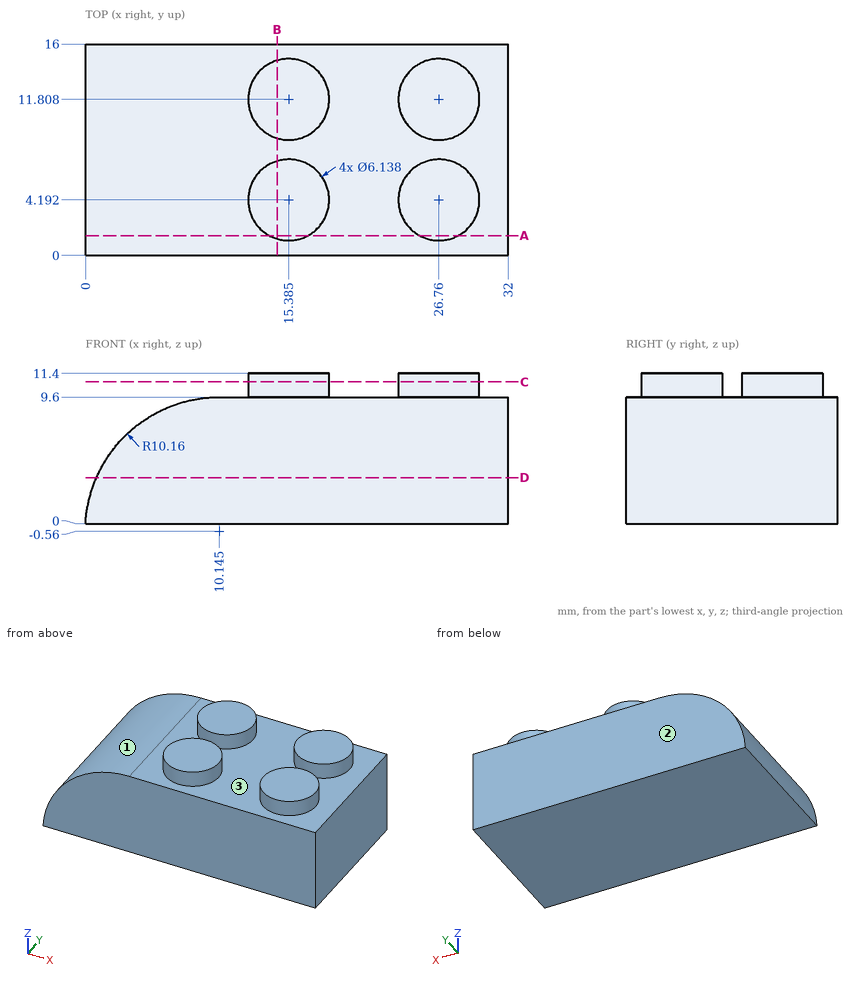
Design review of the part shown in the three views and the two pictorial views. Dimensions are in mm from the part's minimum x, y and z. Coordinates: 2 decimals unless noted, no trailing zeros. Write each loop counter-clockwise with the first axis right and the second up, starting at its lowest first coordinate (ties: lowest second). Pieces come first, ordered by that corner, then holes. Notation, with made-up numbers: (27, 87.25) -> (36, 87.25) arc R25 ccw to (36, 108.25) -> close; hole circle Ø10 at (-35, 82). An arc over 180 degrees is marked (long way). Answer in a Markdown table with one row per item.
1. Wall thickness on probe 1 along Z at (x, y) = (30, 7.5); probe 2 along Y at (x, z) = (26, 10) (1 decimal); probe 3 along X at (y, z) = (8.75, 6) (1 decimal): over which ranges is each line inside the solid? List them lowest first. Write a range as [from, to].
Answers below:
| item | result |
|---|---|
| probe 1 | z = [0, 9.6] |
| probe 2 | y = [1.2, 7.2], [8.8, 14.8] |
| probe 3 | x = [2.4, 32] |
2. Draft analysis for pull direction X (two halves, no side actions). For the marked faces 1, 2 and 3, state which applies: +X half, -X half, draft (parallel to the pull), parting line (faces both ways), or undercut.
Answers below:
| item | result |
|---|---|
| face 1 | -X half |
| face 2 | draft |
| face 3 | undercut |
3. We need section C-C, the plane z = 10.75. State the section outline as (x, y) points (1 decimal).
Answers below:
| item | result |
|---|---|
| outline | circle Ø6.1 at (15.4, 4.2); circle Ø6.1 at (15.4, 11.8); circle Ø6.1 at (26.8, 4.2); circle Ø6.1 at (26.8, 11.8) |
4. We need section D-D, the plane z = 3.5. State the section outline as (x, y) points, and give its area (3 significant figures).
Answers below:
| item | result |
|---|---|
| outline | (0.83, 0) -> (32, 0) -> (32, 16) -> (0.83, 16) -> close |
| area | 499 mm^2 |
5. We need section B-B, the plane x = 14.5. State the section outline as (y, z) points.
Answers below:
| item | result |
|---|---|
| outline | (0, 0) -> (16, 0) -> (16, 9.6) -> (14.75, 9.6) -> (14.75, 11.4) -> (8.87, 11.4) -> (8.87, 9.6) -> (7.13, 9.6) -> (7.13, 11.4) -> (1.25, 11.4) -> (1.25, 9.6) -> (0, 9.6) -> close |
6. We need section A-A, the plane y = 1.5. State the section outline as (x, z) points (1 decimal), and give its area (3 significant figures).
Answers below:
| item | result |
|---|---|
| outline | (0, 0) -> (32, 0) -> (32, 9.6) -> (28.2, 9.6) -> (28.2, 11.4) -> (25.3, 11.4) -> (25.3, 9.6) -> (16.9, 9.6) -> (16.9, 11.4) -> (13.9, 11.4) -> (13.9, 9.6) -> (10.1, 9.6) arc R10.2 ccw to start |
| area | 296 mm^2 |
